from build123d import *

# Parameters (mm, degrees)
SKETCH_1_R      = 12.4
EXTRUDE_1_DEPTH = 3


with BuildPart() as part:
    # 草圖1 → 填料-伸長1 (new body)
    with BuildSketch(Plane(origin=(0, 0, 0), x_dir=(1, 0, 0), z_dir=(0, 1, 0))):
        Polygon((0, 76.568542495), (0, 20), (20, 0), (76.568542495, 0), align=None)
        with Locations(Location((24.142135624, 24.142135624, 0), (0, 0, 270))):
            Circle(SKETCH_1_R, mode=Mode.SUBTRACT)
    extrude(amount=EXTRUDE_1_DEPTH)


solid = part.part
Verification items for the finished model (mm, model axes). Give positions to 0.01 mm unless a question says otherwise; leave off trailing zeros. Write each loop counter-clockwise with the first axis right and the second up, starting at its lowest first coordinate (ties: lowest second). Pieces come first, ordered by that corner, then holes. Notation, with made-up numbers: M 54,28.25 L 105,28.25 A16 ccw 105,50.25 Z; hole C 24.25,23 d9. An arc over 180 degrees is marked long. Use CSV: the item, a comma, the result in double quotes.
1) Cross-section at A-A (x = 29). Enter the section's corners in (y, z).
Final values:
outline,"M 0,-47.57 L 3,-47.57 L 3,-35.55 L 0,-35.55 Z; M 0,-12.73 L 3,-12.73 L 3,0 L 0,0 Z"
2) Cross-section at B-B (z = -30.5). Enter the section's corners in (x, y), plus the area to 3 significant figures.
Final values:
outline,"M 0,0 L 13.5,0 L 13.5,3 L 0,3 Z; M 34.79,0 L 46.07,0 L 46.07,3 L 34.79,3 Z"
area,"74.3 mm²"
3) Cross-section at D-D (x = 66). Enter the section's corners in (y, z).
Final values:
outline,"M 0,-10.57 L 3,-10.57 L 3,0 L 0,0 Z"
4) Go/stop test with a flat-tipped pin: pin 1 Ø1 at (x, y) = (10, 1.5) entering from -Z. Record where the tip stops, or that it passes through.
Final values:
pin 1,"z = -67.07"
5) Release check for a two-part mould opening along Z. For faces 1 (the face through (38.82, 1.48, -37.75)), 2 (the face through (48, 1, 0)), 3 (the face through (35.3, 3, -30)), 4 (the face through (13.14, 1.48, -18.42)) record: released by +Z, released by -Z, zero draft, split by the parting line, or undercut.
Final values:
face 1,"released by -Z"
face 2,"released by +Z"
face 3,"zero draft"
face 4,"undercut"
6) Cross-section at C-C (y = 0.9). Enter the section's corners in (x, z), plus the area to 3 significant figures.
Final values:
outline,"M 0,-76.57 L 76.57,0 L 20,0 L 0,-20 Z; hole C 24.14,-24.14 d24.8"
area,"2,250 mm²"
7) Material ranges on line 1 along Z through (x, y) = (14.5, 1.75); line 2 along X through (y, z) = (2.2, -16); line 3 along Z through (x, y) = (23.5, 0.95), recorded low to high.
Final values:
line 1,"-62.07 to -31.94, -16.35 to -5.5"
line 2,"4 to 14.79, 33.49 to 60.57"
line 3,"-53.07 to -36.53, -11.76 to 0"
